Verification items for the finished model (mm, model axes). A direction names the side the tool comes from. Round coordinates to 2 decimals unless told otherwise and drop trailing zeros. Write each loop counter-clockwise with the first axis right and the second up, starting at its lowest first coordinate (ties: lowest second). Pieces come first, ordered by that corner, then holes. Notation, with made-up numbers: (-1.5, 65.5) - (33.5, 65.5) arc R7 ccw to (33.5, 71.5) - close; hole circle Ø3 at (-22.5, 84). An arc over 180 degrees is marked (long way). Write each question's results on one line, items separated by ' | '.
```python
from build123d import *

# Parameters (mm, degrees)
SKIZZE1_W                       = 35
SKIZZE1_H                       = 50
SKIZZE1_R                       = 1.65
AUFSATZ_LINEAR_AUSTRAGEN1_DEPTH = 10.95
SKIZZE2_W                       = 50
SKIZZE2_H                       = 5.5
SCHNITT_LINEAR_AUSTRAGEN1_DEPTH = 9
SKIZZE3_W                       = 35
SKIZZE3_H                       = 7.25
SCHNITT_LINEAR_AUSTRAGEN2_DEPTH = 2


with BuildPart() as part:
    # Skizze1 → Aufsatz-Linear austragen1 (new body)
    with BuildSketch(Plane.XY):
        Rectangle(SKIZZE1_W, SKIZZE1_H)
        with Locations((-8.75, 22)):
            Circle(SKIZZE1_R, mode=Mode.SUBTRACT)
        with Locations((8.75, 22)):
            Circle(SKIZZE1_R, mode=Mode.SUBTRACT)
    extrude(amount=AUFSATZ_LINEAR_AUSTRAGEN1_DEPTH)

    # Skizze2 → Schnitt-Linear austragen1 (cut)
    with BuildSketch(Plane.XY.offset(10.95)):
        with Locations((0, 15)):
            Rectangle(SKIZZE2_W, SKIZZE2_H)
    extrude(amount=-SCHNITT_LINEAR_AUSTRAGEN1_DEPTH, mode=Mode.SUBTRACT)

    # Skizze3 → Schnitt-Linear austragen2 (cut)
    with BuildSketch(Plane.XY.offset(10.95)):
        with Locations((0, 21.375)):
            Rectangle(SKIZZE3_W, SKIZZE3_H)
    extrude(amount=-SCHNITT_LINEAR_AUSTRAGEN2_DEPTH, mode=Mode.SUBTRACT)


solid = part.part
```
(1) Section check B-B (x = -8.75). Record the cut outline in (y, z).
Answer:
outline: (-25, 0) - (20.35, 0) - (20.35, 8.95) - (17.75, 8.95) - (17.75, 1.95) - (12.25, 1.95) - (12.25, 10.95) - (-25, 10.95) - close; (23.65, 0) - (25, 0) - (25, 8.95) - (23.65, 8.95) - close
(2) Section check C-C (y = 22). Record the cut outline in (x, z), plus the area to 3 significant figures.
Answer:
outline: (-17.5, 0) - (-10.4, 0) - (-10.4, 8.95) - (-17.5, 8.95) - close; (-7.1, 0) - (7.1, 0) - (7.1, 8.95) - (-7.1, 8.95) - close; (10.4, 0) - (17.5, 0) - (17.5, 8.95) - (10.4, 8.95) - close | area: 254 mm2
(3) Section check D-D (x = -1). Record the cut outline in (y, z), plus the area to 4 significant figures.
Answer:
outline: (-25, 0) - (25, 0) - (25, 8.95) - (17.75, 8.95) - (17.75, 1.95) - (12.25, 1.95) - (12.25, 10.95) - (-25, 10.95) - close | area: 483.5 mm2
(4) Section check A-A (z = 7.5). Record the cut outline in (x, y), plus the area to 3 significant figures.
Answer:
outline: (-17.5, -25) - (17.5, -25) - (17.5, 12.25) - (-17.5, 12.25) - close; (-17.5, 17.75) - (17.5, 17.75) - (17.5, 25) - (-17.5, 25) - close; hole circle Ø3.3 at (-8.75, 22); hole circle Ø3.3 at (8.75, 22) | area: 1,540 mm2
(5) Mould release check, pull along Y, two halves, no side actions. Record for faces 1 (the flat face through (0, 15, 1.95)), 2 (the flat face through (0, 0, 0)), 3 (the flat face through (0, -25, 5)): released by +Y, released by -Y, zero draft, split by the parting line, or undercut.
Answer:
face 1: undercut | face 2: zero draft | face 3: released by -Y
(6) Set-up check for faces 4 (the flat face through (0, 12.25, 7)), 5 (the flat face through (0, -6, 10.95)), 6 (the flat face through (0, 21, 8.95)): record each of +Z, -Z, +X, -X, +Y, -Y from which the full face is reachable in a straight line by a thin tool's end or side.
Answer:
face 4: +Z, +X, -X | face 5: +Z, +X, -X, +Y, -Y | face 6: +Z, +X, -X, +Y
(7) Thickness scan on L1, parallel to Y at x = 8.75, z = 3.5; L2, parallel to X at y = 22, z = 2.75; L3, parallel to Y at x = 2, z = 2. Record the ranges inside material, lowest first.
Answer:
L1: -25 to 12.25, 17.75 to 20.35, 23.65 to 25 | L2: -17.5 to -10.4, -7.1 to 7.1, 10.4 to 17.5 | L3: -25 to 12.25, 17.75 to 25
(8) Go/stop test with flat-tipped pins: pin 1 Ø2 at (x, y) = (14, -11) entering from -Z; pin 2 Ø3 at (x, y) = (-3, 16.5) entering from +Z. Record where each tip stops, or that it passes through.
Answer:
pin 1: z = 0 | pin 2: z = 8.95
